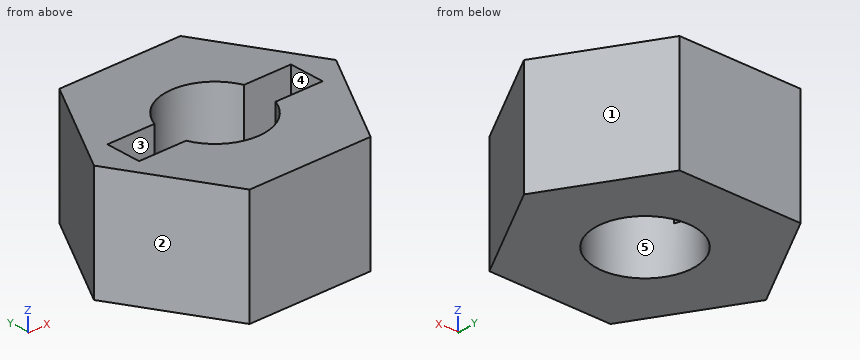
```python
from build123d import *

# Parameters (mm, degrees)
F0_R     = 2.75
F1_DEPTH = 6.5
F3_DEPTH = 4


with BuildPart() as f1:
    # F0 (on Top) → F1 (new body)
    with BuildSketch(Plane.XY):
        Polygon((3.4686009319, -5.997400068), (6.9282012815, 0.0051964886), (3.4596003496, 6.0025965566), (-3.4686009319, 5.997400068), (-6.9282012815, -0.0051964886), (-3.4596003496, -6.0025965566), align=None)
        Circle(F0_R, mode=Mode.SUBTRACT)
    extrude(amount=F1_DEPTH)

    # F2 (on face) → F3 (cut)
    with BuildSketch(Plane.XY.offset(6.5)):
        with BuildLine():
            Line((-5.25, -1), (-2.5617376915, -1))
            ThreePointArc((-2.5617376915, -1), (-2.75, 0), (-2.5617376915, 1))
            Line((-2.5617376915, 1), (-5.25, 1))
            Line((-5.25, 1), (-5.25, -1))
        make_face()
        with BuildLine():
            Line((2.5617376915, -1), (5.25, -1))
            Line((5.25, -1), (5.25, 1))
            Line((5.25, 1), (2.5617376915, 1))
            ThreePointArc((2.5617376915, 1), (2.7025246208, 0.5087835239), (2.75, 0))
            ThreePointArc((2.75, 0), (2.7025246208, -0.5087835239), (2.5617376915, -1))
        make_face()
    extrude(amount=-F3_DEPTH, mode=Mode.SUBTRACT)


solid = f1.part
```
For this review, take the finished solid that the model builds, in its own axes (mm). Face numbers are marked on the shaded views. A direction names the side the tool comes from. Round coordinates to 2 decimals unless told otherwise and drop trailing zeros. Loops run counter-clockwise (first coordinate to the right, second up) from the corner with the lowest first, then second, coordinate; pieces in that order, holes last.
(1) We need section C-C (x = 4.75). Give the boundary of the cut face in (y, z).
Returned:
outline: (-3.77, 0) - (3.77, 0) - (3.77, 6.5) - (1, 6.5) - (1, 2.5) - (-1, 2.5) - (-1, 6.5) - (-3.77, 6.5) - close
(2) We need section B-B (z = 2.25). Give the boundary of the cut face in (x, y), plus the area to 3 significant figures.
Returned:
outline: (-6.93, -0.01) - (-3.46, -6) - (3.47, -6) - (6.93, 0.01) - (3.46, 6) - (-3.47, 6) - close; hole circle Ø5.5 at (0, 0)
area: 101 mm2
(3) We need section A-A (x = 0). Give the boundary of the cut face in (y, z).
Returned:
outline: (-6, 0) - (-2.75, 0) - (-2.75, 6.5) - (-6, 6.5) - close; (2.75, 0) - (6, 0) - (6, 6.5) - (2.75, 6.5) - close
(4) We need section D-D (z = 5.25). Give the boundary of the cut face in (x, y), plus the area to 3 significant figures.
Returned:
outline: (-6.93, -0.01) - (-3.46, -6) - (3.47, -6) - (6.93, 0.01) - (3.46, 6) - (-3.47, 6) - close; hole (-5.25, -1) - (-2.56, -1) arc R2.75 ccw to (2.56, -1) - (5.25, -1) - (5.25, 1) - (2.56, 1) arc R2.75 ccw to (-2.56, 1) - (-5.25, 1) - close
area: 90.7 mm2
(5) Mouldability with a two-part tool opening along X and no side actions: class the marked faces 1, 2 and 3 as released by +X, released by -X, zero draft, split by the parting line, or undercut.
Returned:
face 1: released by +X
face 2: released by -X
face 3: undercut
(6) Wall thickness on line 1 along Y through (x, z) = (1, 4.5); line 2 along Y through (x, z) = (0, 3); line 3 along X through (y, z) = (0.5, 4.25): over which ranges is each line inside the solid? List them lowest first.
Returned:
line 1: y = -6 to -2.56, 2.56 to 6
line 2: y = -6 to -2.75, 2.75 to 6
line 3: x = -6.64 to -5.25, 5.25 to 6.64
(7) Clearance check with flat-ended pins moving along their axes: P1, Ø1.6, axis at x = -4, y = 0, coming from the +Z side; P2, Ø2, axis at y = 3, z = 1.5, coming from the -X side; P3, Ø1.3, axis at x = 4.5, z = 4, coming from the -Y side. State where each tip first meets the part, or that it passes through.
Returned:
P1: stops at z = 2.5
P2: stops at x = -5.77
P3: stops at y = -5.34
(8) Tool access review of the marked faces 4 and 5: name each direction out of +Z, -Z, +X, -X, +Y, -Y from which nothing blocks a thin tool from reaching the whole face with its end or side.
Returned:
face 4: +Z
face 5: +Z, -Z
